Check sheet for the drawn part. Datum: minimum x, y, z corner. Units: mm. A direction names the side the tool comes from. Give positions to 0.01 mm unless a question says otherwise; leave off trailing zeros. Order: outer loops, then holes, each group sorted by start corner. A loop starts at its lowest first (then second) coordinate and runs counter-clockwise, first axis right, second up.
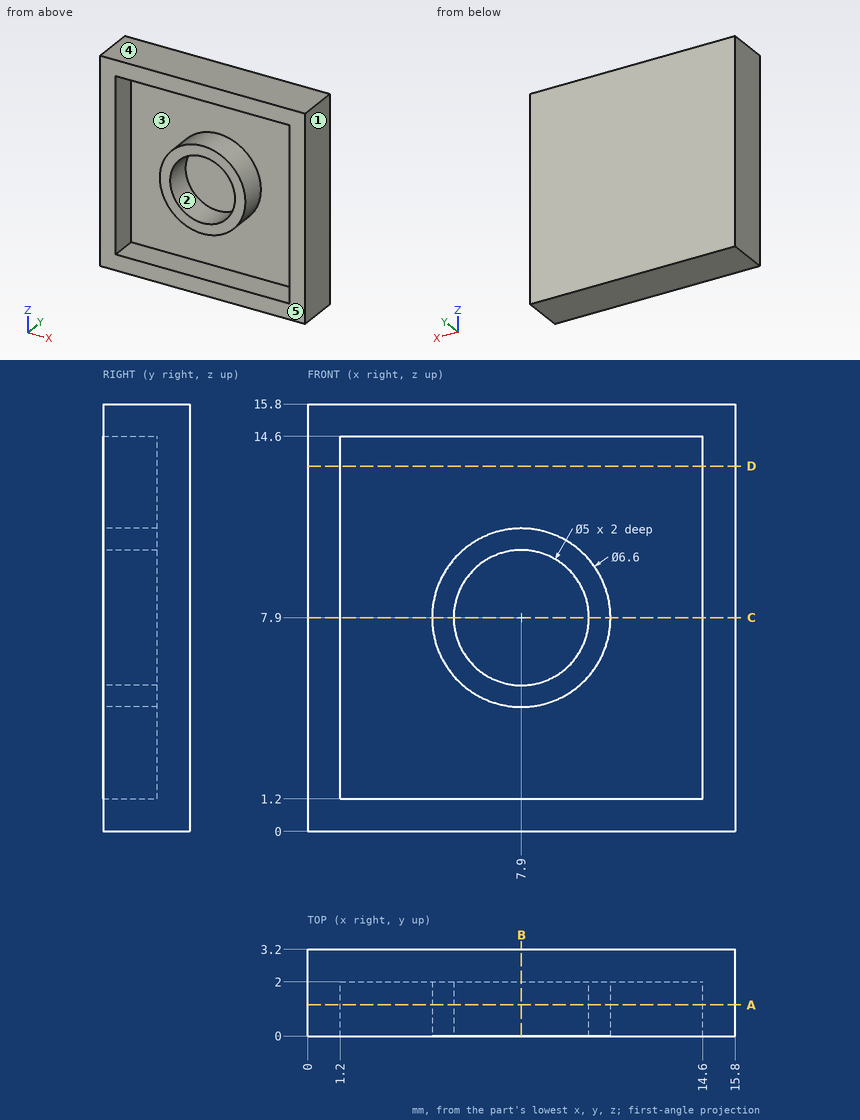
(1) Section check B-B, the plane x = 7.9. Enter the section's corners in (y, z).
Solved:
outline: (0, 0) - (3.2, 0) - (3.2, 15.8) - (0, 15.8) - (0, 14.6) - (2, 14.6) - (2, 11.2) - (0, 11.2) - (0, 10.4) - (2, 10.4) - (2, 5.4) - (0, 5.4) - (0, 4.6) - (2, 4.6) - (2, 1.2) - (0, 1.2) - close
(2) Section check D-D, the plane z = 13.5. Enter the section's corners in (x, y), then the cut area to 3 significant figures.
Solved:
outline: (0, 0) - (1.2, 0) - (1.2, 2) - (14.6, 2) - (14.6, 0) - (15.8, 0) - (15.8, 3.2) - (0, 3.2) - close
area: 23.8 mm2
(3) Scan lines: line 1 (Z direction, x = 7.9, y = 0.4); line 2 (X direction, y = 1, z = 12.75); line 3 (Y direction, x = 13.5, z = 7.75). Record each from-to range of solid material in increasing order.
Solved:
line 1: z = 0 to 1.2, 4.6 to 5.4, 10.4 to 11.2, 14.6 to 15.8
line 2: x = 0 to 1.2, 14.6 to 15.8
line 3: y = 2 to 3.2
(4) Set-up check for the marked faces 1 and 2: record each of +Z, -Z, +X, -X, +Y, -Y from which the full face is reachable in a straight line by a thin tool's end or side.
Solved:
face 1: +Z, -Z, +X, +Y, -Y
face 2: -Y
(5) Go/stop test with a flat-tipped pin: pin 1 (1.6 mm diameter, centred on y = 1, z = 6, fed in from -X). Record where the tip stops, or that it passes through.
Solved:
pin 1: stops at x = 0
(6) Release check for a two-part mould opening along Z. For the marked faces 3, 4 and 5 record: pulls with the +Z half, pulls with the -Z half, needs draft (parallel to the pull), parting line crosses it, or undercut.
Solved:
face 3: undercut
face 4: pulls with the +Z half
face 5: needs draft
(7) Section check A-A, the plane y = 1.15. Enter the section's corners in (x, z).
Solved:
outline: (0, 0) - (15.8, 0) - (15.8, 15.8) - (0, 15.8) - close; circle Ø6.6 at (7.9, 7.9); hole (1.2, 1.2) - (14.6, 1.2) - (14.6, 14.6) - (1.2, 14.6) - close; hole circle Ø5 at (7.9, 7.9)
(8) Section check C-C, the plane z = 7.9. Enter the section's corners in (x, y).
Solved:
outline: (0, 0) - (1.2, 0) - (1.2, 2) - (4.6, 2) - (4.6, 0) - (5.4, 0) - (5.4, 2) - (10.4, 2) - (10.4, 0) - (11.2, 0) - (11.2, 2) - (14.6, 2) - (14.6, 0) - (15.8, 0) - (15.8, 3.2) - (0, 3.2) - close
